The listing builds one solid part. Answer for the finished solid, in the listing's coordinates (mm). A direction names the side the tool comes from. Give positions to 0.01 mm unless a question says otherwise; leave off trailing zeros. Loops run counter-clockwise (first coordinate to the right, second up) from the corner with the lowest first, then second, coordinate; pieces in that order, holes last.
Item 1: Consider line 1 along Z through (x, y) = (85.5, 3); line 2 along Y through (x, z) = (206.5, 12.25); line 3 along Y through (x, z) = (143, 23.5). Determine where each line is inside the solid, lowest interval first.
Item 2: Section A-A, the plane x = -21.5 is taken. Give the vertices of the cut face in (y, z), and give its area (3 significant figures).
Item 3: This flat-tipped pin is pushed along its axis until it touches: pin 1 Ø3 at (x, y) = (193.49, 0) entering from -Z. Where does it stop, or does it pass through?
Item 4: A tool of negligible diameter and unlimited length cuts with its end or side. For faces 1 (the face through (26, 12.7, 13)), 2 (the face through (26, 0, 2.54)), from which of +Z, -Z, +X, -X, +Y, -Y can it reach the whole face along a straight path? Write none if from no direction.
Item 5: The mould has two halves that part along Z. Classify faces 3 (the face through (26, 10.16, 13)), 4 (the face through (26, 0, 0)), 5 (the face through (-249.338, 11, 13)): pulls with the +Z half, pulls with the -Z half, needs draft (parallel to the pull), parting line crosses it, or undercut.
from build123d import *

# Parameters (mm, degrees)
F0_W     = 558.8
F0_H     = 25.4
F0_R     = 2.5527
F1_DEPTH = 25.4
F2_W     = 20.32
F2_H     = 20.32
F3_DEPTH = 508
F5_D     = 5.1054
F6_W     = 20.32
F6_H     = 20.32
F7_DEPTH = 558.8


with BuildPart() as f1:
    # F0 (on Top) → F1 (new body)
    with BuildSketch(Plane.XY):
        with Locations((30.061689, 0)):
            Rectangle(F0_W, F0_H)
        with Locations((-238.314838, 0)):
            Circle(F0_R, mode=Mode.SUBTRACT)
        with Locations((-212.914838, 0)):
            Circle(F0_R, mode=Mode.SUBTRACT)
        with Locations((-187.514838, 0)):
            Circle(F0_R, mode=Mode.SUBTRACT)
        with Locations((-162.114838, 0)):
            Circle(F0_R, mode=Mode.SUBTRACT)
        with Locations((-136.714838, 0)):
            Circle(F0_R, mode=Mode.SUBTRACT)
        with Locations((-111.314838, 0)):
            Circle(F0_R, mode=Mode.SUBTRACT)
        with Locations((-85.914838, 0)):
            Circle(F0_R, mode=Mode.SUBTRACT)
        with Locations((-60.514838, 0)):
            Circle(F0_R, mode=Mode.SUBTRACT)
        with Locations((-35.114838, 0)):
            Circle(F0_R, mode=Mode.SUBTRACT)
        with Locations((-9.714838, 0)):
            Circle(F0_R, mode=Mode.SUBTRACT)
        with Locations((15.685162, 0)):
            Circle(F0_R, mode=Mode.SUBTRACT)
        with Locations((41.085162, 0)):
            Circle(F0_R, mode=Mode.SUBTRACT)
        with Locations((66.485162, 0)):
            Circle(F0_R, mode=Mode.SUBTRACT)
        with Locations((91.885162, 0)):
            Circle(F0_R, mode=Mode.SUBTRACT)
        with Locations((117.285162, 0)):
            Circle(F0_R, mode=Mode.SUBTRACT)
        with Locations((142.685162, 0)):
            Circle(F0_R, mode=Mode.SUBTRACT)
        with Locations((168.085162, 0)):
            Circle(F0_R, mode=Mode.SUBTRACT)
        with Locations((193.485162, 0)):
            Circle(F0_R, mode=Mode.SUBTRACT)
        with Locations((218.885162, 0)):
            Circle(F0_R, mode=Mode.SUBTRACT)
        with Locations((244.285162, 0)):
            Circle(F0_R, mode=Mode.SUBTRACT)
        with Locations((269.685162, 0)):
            Circle(F0_R, mode=Mode.SUBTRACT)
        with Locations((295.085162, 0)):
            Circle(F0_R, mode=Mode.SUBTRACT)
    extrude(amount=F1_DEPTH)

    # F2 (on face) → F3 (cut)
    with BuildSketch(Plane(origin=(-249.338311, 0, 0), x_dir=(0, -1, 0), z_dir=(-1, 0, 0))):
        with Locations((0, 12.7)):
            Rectangle(F2_W, F2_H)
    extrude(amount=-F3_DEPTH, mode=Mode.SUBTRACT)

    # F5 (through all)
    with Locations(Plane.XZ.offset(12.7)):
        with Locations((118.961689, 12.7), (220.561689, 12.7), (42.761689, 12.7), (169.761689, 12.7), (271.361689, 12.7), (-33.438311, 12.7), (195.161689, 12.7), (245.961689, 12.7), (-58.838311, 12.7), (-84.238311, 12.7), (-185.838311, 12.7), (-236.638311, 12.7), (17.361689, 12.7), (-8.038311, 12.7), (296.761689, 12.7), (68.161689, 12.7), (93.561689, 12.7), (144.361689, 12.7), (-211.238311, 12.7), (-109.638311, 12.7), (-135.038311, 12.7), (-160.438311, 12.7)):
            Hole(F5_D / 2)

    # F6 (on face) → F7 (cut)
    with BuildSketch(Plane.YZ.offset(309.461689)):
        with Locations((0, 12.7)):
            Rectangle(F6_W, F6_H)
    extrude(amount=-F7_DEPTH, mode=Mode.SUBTRACT)


solid = f1.part
Worked answers:
1. line 1: z = 0 to 2.54, 22.86 to 25.4
1. line 2: y = -12.7 to -10.16, 10.16 to 12.7
1. line 3: y = -12.7 to -2.53, 2.53 to 12.7
2. outline: (-12.7, 0) - (12.7, 0) - (12.7, 25.4) - (-12.7, 25.4) - close; hole (-10.16, 2.54) - (10.16, 2.54) - (10.16, 22.86) - (-10.16, 22.86) - close
2. area: 232 mm2
3. pin 1: passes through
4. face 1: +Z, -Z, +X, -X, +Y
4. face 2: +X, -X
5. face 3: undercut
5. face 4: pulls with the -Z half
5. face 5: needs draft
